Part print with two shaded views. Sizes in mm from the minimum x, y, z corner. Round coordinates to 2 decimals unless told otherwise and drop trailing zeros. Write each loop counter-clockwise with the first axis right and the second up, starting at its lowest first coordinate (ties: lowest second). Pieces come first, ordered by that corner, then holes. Notation, with made-up numbers: (-7.5, 39) - (51.5, 39) arc R20 cw to (51.5, 78) - close; hole circle Ø1 at (-11, 40.5). An arc over 180 degrees is marked (long way). Answer as a JSON object with one key per item and string values. Group by question number.
Item 1: Slice it at B-B, the plane z = 2.3. List the corners of the cut face in (x, y).
Item 2: Slice it at A-A, the plane x = 8. List the corners of the cut face in (y, z), then the cut area to 3 significant figures.
Item 3: Flat gauge pin, fed straight in: pin 1 (1 mm diameter, centred on x = 11.5, y = 10, fed in from -Z). Where does the tip first touch, or does it go through?
Item 4: Probe line 1 (Y direction, x = 68, z = 1.55); line 2 (X direction, y = 9, z = 1.1); line 3 (X direction, y = 13, z = 0.9). List the from-to ranges inside material, lowest first. Write a range as from..to.
Item 5: Slice it at C-C, the plane y = 10. List the corners of the cut face in (x, z).
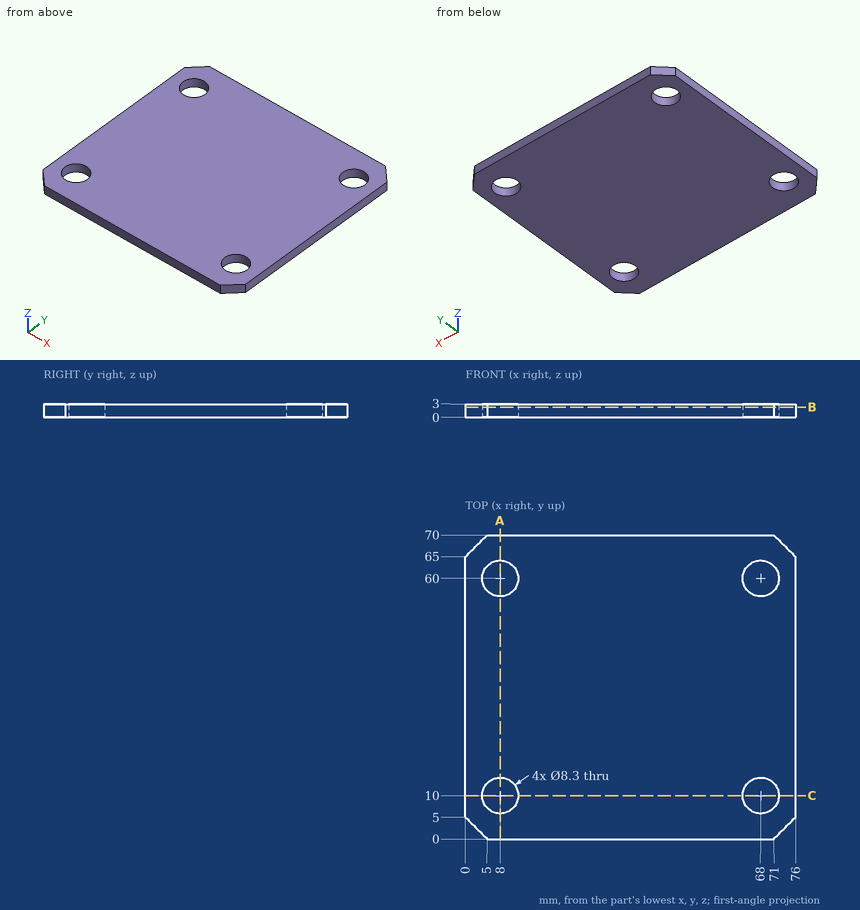
Geometry says:
{
 "1": {"outline": "(0, 5) - (5, 0) - (71, 0) - (76, 5) - (76, 65) - (71, 70) - (5, 70) - (0, 65) - close; hole circle Ø8.3 at (8, 10); hole circle Ø8.3 at (8, 60); hole circle Ø8.3 at (68, 10); hole circle Ø8.3 at (68, 60)"},
 "2": {"outline": "(0, 0) - (5.85, 0) - (5.85, 3) - (0, 3) - close; (14.15, 0) - (55.85, 0) - (55.85, 3) - (14.15, 3) - close; (64.15, 0) - (70, 0) - (70, 3) - (64.15, 3) - close", "area": "160 mm^2"},
 "3": {"pin 1": "passes through"},
 "4": {"line 1": "y = 0..5.85, 14.15..55.85, 64.15..70", "line 2": "x = 0..3.97, 12.03..63.97, 72.03..76", "line 3": "x = 0..5.13, 10.87..65.13, 70.87..76"},
 "5": {"outline": "(0, 0) - (3.85, 0) - (3.85, 3) - (0, 3) - close; (12.15, 0) - (63.85, 0) - (63.85, 3) - (12.15, 3) - close; (72.15, 0) - (76, 0) - (76, 3) - (72.15, 3) - close"}
}
